Geometry check sheet. Reference: the model listing, model coordinates, mm. Face numbers are marked on the shaded views. A direction names the side the tool comes from. Give positions to 0.01 mm unless a question says otherwise; leave off trailing zeros. Loops run counter-clockwise (first coordinate to the right, second up) from the corner with the lowest first, then second, coordinate; pieces in that order, holes last. Notation, with made-up numbers: (-19.75, -4.75) -> (28.25, -4.75) arc R21 cw to (28.25, 9.25) -> close; hole circle Ø8 at (-2.5, -25.75). An arc over 180 degrees is marked (long way). Write item = value, one per line. Start each with the question number.
```python
from build123d import *

# Parameters (mm, degrees)
SKETCH1_W               = 15
SKETCH1_H               = 10
BOSS_EXTRUDE1_DEPTH     = 10
SKETCH2_W               = 15
SKETCH2_H               = 10
SKETCH2_W_2             = 12.8
SKETCH2_H_2             = 7.8
CUT_EXTRUDE1_DEPTH      = 8.4
CHAMFER1_SIZE           = 1
CHAMFER1_SIZE2          = 1.732050808
CHAMFER1_PART_2_SIZE    = 1
CHAMFER1_PART_2_SIZE2   = 1.732050808
CHAMFER1_PART_3_SIZE    = 1
CHAMFER1_PART_3_SIZE2   = 1.732050808
CHAMFER1_PART_4_SIZE    = 1
CHAMFER1_PART_4_SIZE2   = 1.732050808
SKETCH3_W               = 0.5
SKETCH3_H               = 4
EXTRUDE_THIN1_DEPTH     = 6.6
FILLET1_R               = 1
SKETCH4_R               = 0.5
CUT_EXTRUDE2_DEPTH      = 6.6
SKETCH5_W               = 11.535898384
SKETCH5_H               = 6.535898384
BOSS_EXTRUDE2_DEPTH     = 2.5
CUT_EXTRUDE5_DEPTH      = 2.732050808
CUT_EXTRUDE5_DEPTH_BACK = 7.5


with BuildPart() as part:
    # Sketch1 → Boss-Extrude1 (new body)
    with BuildSketch(Plane(origin=(0, 0, 0), x_dir=(1, 0, 0), z_dir=(0, 1, 0))):
        Rectangle(SKETCH1_W, SKETCH1_H)
    extrude(amount=BOSS_EXTRUDE1_DEPTH)

    # Sketch2 → Cut-Extrude1 (cut)
    with BuildSketch(Plane.XZ):
        Rectangle(SKETCH2_W, SKETCH2_H)
        Rectangle(SKETCH2_W_2, SKETCH2_H_2, mode=Mode.SUBTRACT)
    extrude(amount=-CUT_EXTRUDE1_DEPTH, mode=Mode.SUBTRACT)

    # Chamfer1
    chamfer1_edges = [part.edges().sort_by_distance(p)[0] for p in [
        (-7.5, 10, 0),
    ]]
    chamfer1_side = [part.faces().sort_by_distance(p)[0] for p in [
        (-7.5, 9.2, 0),
    ]]
    chamfer(chamfer1_edges, length=CHAMFER1_SIZE, length2=CHAMFER1_SIZE2, reference=chamfer1_side[0])

    # Chamfer1 part 2
    chamfer1_part_2_edges = [part.edges().sort_by_distance(p)[0] for p in [
        (0, 10, 5),
    ]]
    chamfer1_part_2_side = [part.faces().sort_by_distance(p)[0] for p in [
        (0, 9.2, 5),
    ]]
    chamfer(chamfer1_part_2_edges, length=CHAMFER1_PART_2_SIZE, length2=CHAMFER1_PART_2_SIZE2, reference=chamfer1_part_2_side[0])

    # Chamfer1 part 3
    chamfer1_part_3_edges = [part.edges().sort_by_distance(p)[0] for p in [
        (7.5, 10, 0),
    ]]
    chamfer1_part_3_side = [part.faces().sort_by_distance(p)[0] for p in [
        (7.5, 9.2, 0),
    ]]
    chamfer(chamfer1_part_3_edges, length=CHAMFER1_PART_3_SIZE, length2=CHAMFER1_PART_3_SIZE2, reference=chamfer1_part_3_side[0])

    # Chamfer1 part 4
    chamfer1_part_4_edges = [part.edges().sort_by_distance(p)[0] for p in [
        (0, 10, -5),
    ]]
    chamfer1_part_4_side = [part.faces().sort_by_distance(p)[0] for p in [
        (0, 9.2, -5),
    ]]
    chamfer(chamfer1_part_4_edges, length=CHAMFER1_PART_4_SIZE, length2=CHAMFER1_PART_4_SIZE2, reference=chamfer1_part_4_side[0])

    # Sketch3 → Extrude-Thin1 (add)
    with BuildSketch(Plane.XZ):
        with Locations((3.65, 0)):
            Rectangle(SKETCH3_W, SKETCH3_H)
        with Locations((0.65, 0)):
            Rectangle(SKETCH3_W, SKETCH3_H)
    extrude(amount=EXTRUDE_THIN1_DEPTH)

    # Fillet1
    fillet1_edges = [part.edges().sort_by_distance(p)[0] for p in [
        (3.65, -6.6, 2),
        (3.65, -6.6, -2),
        (0.65, -6.6, 2),
        (0.65, -6.6, -2),
    ]]
    fillet(fillet1_edges, radius=FILLET1_R)

    # Sketch4 → Cut-Extrude2 (cut)
    with BuildSketch(Plane.ZY.offset(-0.4)):
        with Locations((0, -5.6)):
            Circle(SKETCH4_R)
    extrude(amount=-CUT_EXTRUDE2_DEPTH, mode=Mode.SUBTRACT)

    # Sketch5 → Boss-Extrude2 (add)
    with BuildSketch(Plane(origin=(0, 10, 0), x_dir=(1, 0, 0), z_dir=(0, 1, 0))):
        Rectangle(SKETCH5_W, SKETCH5_H)
    extrude(amount=BOSS_EXTRUDE2_DEPTH)

    # Sketch6 → Cut-Extrude5 (cut, two sides)
    with BuildSketch(Plane.XY.offset(3.267949192)) as cut_extrude5_sk:
        with BuildLine():
            Line((57.587759611, 35.04655449), (5.767949192, 12.5))
            ThreePointArc((5.767949192, 12.5), (0.123547764, 10.713329317), (-5.767949192, 10.128758351))
            Line((-5.767949192, 10.128758351), (-62.279560483, 10.40743474))
            Line((-62.279560483, 10.40743474), (-85.036348275, 121.117362453))
            Line((-85.036348275, 121.117362453), (34.83097182, 145.756482204))
            Line((34.83097182, 145.756482204), (57.587759611, 35.04655449))
        make_face()
    extrude(amount=CUT_EXTRUDE5_DEPTH, mode=Mode.SUBTRACT)
    extrude(cut_extrude5_sk.sketch, amount=-CUT_EXTRUDE5_DEPTH_BACK, mode=Mode.SUBTRACT)


solid = part.part
```
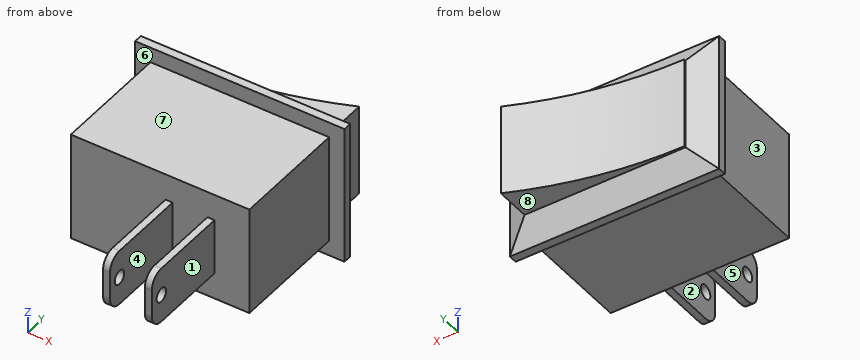
1) Section check B-B (z = 0). Enter the section's corners in (x, y), plus the area to 3 significant figures.
2) Depth check by flat-ended pin: pin 1 Ø4 at (y, z) = (4, 1) entering from -X; pin 2 Ø1.5 at (x, z) = (-5, -3) entering from +Y; pin 3 Ø4 at (y, z) = (4, 3) entering from +X. Enter the tip coordinate at first touch or a pass-through.
3) Section check C-C (x = 5). Enter the section's corners in (y, z).
4) Thickness scan on line 1 (X direction, y = 0.25, z = 0.75); line 2 (Z direction, x = 2.5, y = 2.5); line 3 (Y direction, x = 3.55, z = 0). Record the ranges inside material, lowest first.
5) Section check A-A (y = -1). Enter the section's corners in (x, z).
6) Tool access check on the marked faces 4, 5, 6, 7 and 8. Record the directions out of +Z, -Z, +X, -X, +Y, -Y that give a thin tool (end or side, any length) a straight path to the whole face; none if there is none.
7) Section check D-D (z = 1.75). Enter the section's corners in (x, y).
8) Draft check along X on the marked faces 1, 2 and 3. Enter one of: released by +X, released by -X, zero draft, split by the parting line, or undercut.
Check result:
q1.outline = (-7.5, 8.4) -> (-6.4, 8.4) -> (-6.4, 0) -> (0.4, 0) -> (0.4, -5.1) -> (0.9, -5.1) -> (0.9, 0) -> (3.4, 0) -> (3.4, -5.1) -> (3.9, -5.1) -> (3.9, 0) -> (6.4, 0) -> (6.4, 8.4) -> (7.5, 8.4) -> (7.5, 9) -> (5.77, 10) -> (5.77, 12.5) arc R28.56 cw to (-5.77, 10.13) -> (-5.77, 10) -> (-7.5, 9) -> close; (0.4, -6.6) -> (0.9, -6.6) -> (0.9, -6.1) -> (0.4, -6.1) -> close; (3.4, -6.6) -> (3.9, -6.6) -> (3.9, -6.1) -> (3.4, -6.1) -> close
q1.area = 146 mm2
q2.pin_1 = -6.4
q2.pin_2 = 10.16
q2.pin_3 = 6.4
q3.outline = (0, -3.9) -> (8.4, -3.9) -> (8.4, -5) -> (9, -5) -> (10, -3.27) -> (12.18, -3.27) -> (12.18, 3.27) -> (10, 3.27) -> (9, 5) -> (8.4, 5) -> (8.4, 3.9) -> (0, 3.9) -> close
q4.line_1 = -6.4 to 6.4
q4.line_2 = -3.9 to 3.9
q4.line_3 = -6.6 to -6.1, -5.1 to 11.64
q5.outline = (0.4, -2) -> (0.9, -2) -> (0.9, 2) -> (0.4, 2) -> close; (3.4, -2) -> (3.9, -2) -> (3.9, 2) -> (3.4, 2) -> close
q6.face_4 = +Z, -Z, -Y
q6.face_5 = +Z, -Z, -X, -Y
q6.face_6 = -Y
q6.face_7 = +Z, +X, -X, -Y
q6.face_8 = -Z, +X, -X, +Y
q7.outline = (-7.5, 8.4) -> (-6.4, 8.4) -> (-6.4, 0) -> (0.4, 0) -> (0.4, -6.26) -> (0.9, -6.26) -> (0.9, 0) -> (3.4, 0) -> (3.4, -6.26) -> (3.9, -6.26) -> (3.9, 0) -> (6.4, 0) -> (6.4, 8.4) -> (7.5, 8.4) -> (7.5, 9) -> (5.77, 10) -> (5.77, 12.5) arc R28.56 cw to (-5.77, 10.13) -> (-5.77, 10) -> (-7.5, 9) -> close
q8.face_1 = released by +X
q8.face_2 = undercut
q8.face_3 = released by -X
